Geometry check sheet. Reference: the model listing, model coordinates, mm. A direction names the side the tool comes from. Round coordinates to 2 decimals unless told otherwise and drop trailing zeros. Loops run counter-clockwise (first coordinate to the right, second up) from the corner with the lowest first, then second, coordinate; pieces in that order, holes last. Notation, with made-up numbers: (16, 66) - (36, 66) arc R30 cw to (36, 92) - close; hole circle Ø5 at (60, 49.25). An arc over 180 degrees is marked (long way). Write item = value, one per line.
```python
from build123d import *

# Parameters (mm, degrees)
SKETCH1_R                = 6
BOSS_EXTRUDE1_DEPTH      = 104
BOSS_EXTRUDE1_DEPTH_BACK = 16
CUT_EXTRUDE3_START       = -16
SKETCH2_W                = 4
SKETCH2_H                = 5
CUT_EXTRUDE3_DEPTH       = 20
CUT_EXTRUDE3_DEPTH_BACK  = 0.0001
CUT_EXTRUDE4_START       = 104
SKETCH2_2_W              = 4
SKETCH2_2_H              = 5
CUT_EXTRUDE4_DEPTH       = 50
CUT_EXTRUDE6_START       = -16
SKETCH3_W                = 4
SKETCH3_H                = 10
CUT_EXTRUDE6_DEPTH       = 6


with BuildPart() as part:
    # Sketch1 → Boss-Extrude1 (new body, two sides)
    with BuildSketch(Plane(origin=(0, 0, 0), x_dir=(1, 0, 0), z_dir=(0, 1, 0))) as boss_extrude1_sk:
        Circle(SKETCH1_R)
    extrude(amount=BOSS_EXTRUDE1_DEPTH)
    extrude(boss_extrude1_sk.sketch, amount=-BOSS_EXTRUDE1_DEPTH_BACK)

    # Sketch2 → Cut-Extrude3 (cut, two sides)
    with BuildSketch(Plane(origin=(0, 0, 0), x_dir=(1, 0, 0), z_dir=(0, 1, 0)).offset(CUT_EXTRUDE3_START)) as cut_extrude3_sk:
        with Locations((0, -6)):
            Rectangle(SKETCH2_W, SKETCH2_H)
    extrude(amount=CUT_EXTRUDE3_DEPTH, mode=Mode.SUBTRACT)
    extrude(cut_extrude3_sk.sketch, amount=-CUT_EXTRUDE3_DEPTH_BACK, mode=Mode.SUBTRACT)

    # Sketch2<2> → Cut-Extrude4 (cut)
    with BuildSketch(Plane(origin=(0, 0, 0), x_dir=(1, 0, 0), z_dir=(0, 1, 0)).offset(CUT_EXTRUDE4_START)):
        with Locations((0, -6)):
            Rectangle(SKETCH2_2_W, SKETCH2_2_H)
    extrude(amount=-CUT_EXTRUDE4_DEPTH, mode=Mode.SUBTRACT)

    # Sketch3 → Cut-Extrude6 (cut)
    with BuildSketch(Plane(origin=(0, 0, 0), x_dir=(1, 0, 0), z_dir=(0, 1, 0)).offset(CUT_EXTRUDE6_START)):
        with Locations((0, -6)):
            Rectangle(SKETCH3_W, SKETCH3_H)
    extrude(amount=CUT_EXTRUDE6_DEPTH, mode=Mode.SUBTRACT)


solid = part.part
```
(1) Section check C-C (z = 2.5). Enter the section's corners in (x, y).
Answers follow:
outline = (-5.45, -16) - (-2, -16) - (-2, -10) - (2, -10) - (2, -16) - (5.45, -16) - (5.45, 104) - (-5.45, 104) - close
(2) Gauge pin test, flat ends, axial feed: pin 1 (2 mm diameter, centred on x = 3.5, y = -0.5, fed in from -Z); pin 2 (0.6 mm diameter, centred on y = 76, z = 4.5, fed in from -X); pin 3 (1.2 mm diameter, centred on x = -0.5, z = 4.5, fed in from +Y). Record the tip position at first contact, or that the pin passes through.
Answers follow:
pin_1 = -5.45
pin_2 = -4.28
pin_3 = 54
(3) Set-up check for faces 1 (the flat face through (0, 104, 0)), 2 (the flat face through (-2, -8, 4)), 3 (the flat face through (0, 54, 5)): record each of +Z, -Z, +X, -X, +Y, -Y from which the full face is reachable in a straight line by a thin tool's end or side.
Answers follow:
face_1 = +Z, -Z, +X, -X, +Y
face_2 = +Z, -Y
face_3 = +Z, +Y
(4) Section check A-A (x = 0). Enter the section's corners in (y, z).
Answers follow:
outline = (-16, -6) - (104, -6) - (104, 3.5) - (54, 3.5) - (54, 6) - (4, 6) - (4, 3.5) - (-10, 3.5) - (-10, 1) - (-16, 1) - close
(5) Mould release check, pull along Z, two halves, no side actions. Record for faces 4 (the cylindrical face through (-0.78, 44.84, -5.95)), 5 (the flat face through (0, -13, 1)), 6 (the flat face through (2, 79, 5)): pulls with the +Z half, pulls with the -Z half, needs draft (parallel to the pull), parting line crosses it, or undercut.
Answers follow:
face_4 = parting line crosses it
face_5 = pulls with the +Z half
face_6 = needs draft
(6) Section check B-B (y = 88.5). Enter the section's corners in (x, z).
Answers follow:
outline = (-2, 3.5) - (-2, 5.66) arc R6 ccw (long way) to (2, 5.66) - (2, 3.5) - close
(7) Section check D-D (y = 43). Enter the section's corners in (x, z).
Answers follow:
outline = circle Ø12 at (0, 0)
(8) Scan lines: L1, parallel to Y at x = -1.25, z = 2.25; L2, parallel to X at y = 73, z = 0.25; L3, parallel to Z at x = -3.75, y = 37. Record each from-to range of solid material in increasing order. Write a range as [from, to].
Answers follow:
L1 = [-10, 104]
L2 = [-5.99, 5.99]
L3 = [-4.68, 4.68]
